Work out the finished part from the listing and answer in its coordinate system (mm). A direction names the side the tool comes from. Round coordinates to 2 decimals unless told otherwise and drop trailing zeros. Order: outer loops, then holes, each group sorted by start corner. A loop starts at its lowest first (then second) coordinate and runs counter-clockwise, first axis right, second up. Notation, with made-up numbers: (77.25, -25.5) - (88.25, -25.5) arc R10 ccw to (88.25, -13.5) - close; hole circle Ø9 at (-20.75, -26.75). An arc over 180 degrees is marked (long way). Use CSV: the item, a comma, the result in double quotes.
from build123d import *

# Parameters (mm, degrees)
SKETCH_1_W               = 25
SKETCH_1_H               = 16
EXTRUDE_1_DEPTH          = 7
SKETCH_3_W               = 5.9
SKETCH_3_H               = 2.3
FILLET_1_R               = 2
SKETCH_4_R               = 1.75
CUT_EXTRUDE_1_DEPTH      = 37.390245946
CUT_EXTRUDE_2_DEPTH      = 4.5
PATTERN_CIRCULAR_1_COUNT = 18


with BuildPart() as part:
    # 草图1 → 凸台-拉伸1 (new, symmetric)
    with BuildSketch(Plane(origin=(0, 0, 0), x_dir=(1, 0, 0), z_dir=(0, 1, 0))):
        Rectangle(SKETCH_1_W, SKETCH_1_H)
    extrude(amount=EXTRUDE_1_DEPTH, both=True)

    # 草图2 → 旋转1 (revolve)
    with BuildSketch(Plane(origin=(0, 0, 0), x_dir=(1, 0, 0), z_dir=(0, 1, 0)), mode=Mode.PRIVATE) as revolve_1_sk:
        Polygon((-12.5, 4.975068019), (-18.5, 5.5), (-21.5, 5.5), (-21.5, 4.5), (-22.5, 4.5), (-22.5, 6), (-24, 6), (-24, 3), (-19.5, 3), (-19.5, 2), (-12.5, 2), align=None)
        Polygon((19.5, 2), (12.5, 2), (12.5, 4.975068019), (18.5, 5.5), (21.5, 5.5), (21.5, 4.5), (22.5, 4.5), (22.5, 6), (24, 6), (24, 3), (19.5, 3), align=None)
    revolve(revolve_1_sk.sketch.rotate(Axis((-27.060600163, 0, 0), (1, 0, 0)), 180), axis=Axis((-27.060600163, 0, 0), (1, 0, 0)))

    # 草图3 → 旋转2 (revolve)
    with BuildSketch(Plane(origin=(0, 0, 0), x_dir=(1, 0, 0), z_dir=(0, 1, 0))):
        Polygon((7, 8), (7, 10.5), (6.5, 11), (6.5, 12.5), (4, 12.5), (4, 13.5), (4.4, 13.5), (4.4, 16), (2, 16), (2, 19), (4, 19), (4, 23.5), (0, 23.5), (0, 8), align=None)
        with Locations((2.95, -9.15)):
            Rectangle(SKETCH_3_W, SKETCH_3_H)
    revolve(axis=Axis((0, 0, 30.021655922), (0, 0, -1)))

    # 圆角1
    fillet_1_edges = [part.edges().sort_by_distance(p)[0] for p in [
        (-12.5, 0, -8),
        (12.5, 0, -8),
    ]]
    fillet(fillet_1_edges, radius=FILLET_1_R)

    # 草图4 → 切除-拉伸1 (cut, through all)
    with BuildSketch(Plane(origin=(0, 7, 0), x_dir=(1, 0, 0), z_dir=(0, 1, 0))):
        with Locations(Location((-10, 5.5, 0), (0, 0, 270))):
            Circle(SKETCH_4_R)
        with Locations(Location((10, 5.5, 0), (0, 0, 270))):
            Circle(SKETCH_4_R)
    extrude(amount=-CUT_EXTRUDE_1_DEPTH, mode=Mode.SUBTRACT)

    # 草图5 → 切除-拉伸2 (cut)
    with BuildSketch(Plane(origin=(0, 0, -23.5), x_dir=(-1, 0, 0), z_dir=(0, 0, -1))):
        with BuildLine():
            ThreePointArc((0, 4), (0.352895639, 3.937075737), (0.662294506, 3.756058788))
            ThreePointArc((0.662294506, 3.756058788), (1.01494578, 3.820338434), (1.368080573, 3.758770483))
            ThreePointArc((1.368080573, 3.758770483), (0.694592711, 3.939231012), (0, 4))
        make_face()
    cut_extrude_2 = extrude(amount=-CUT_EXTRUDE_2_DEPTH, mode=Mode.SUBTRACT)

    # 阵列(圆周)1: 切除-拉伸2 ×18 about axis
    pattern_circular_1_axis = Axis((0, 0, 0), (0, 0, 1))
    for i in range(1, PATTERN_CIRCULAR_1_COUNT):
        add(cut_extrude_2.rotate(pattern_circular_1_axis, i * 360 / PATTERN_CIRCULAR_1_COUNT), mode=Mode.SUBTRACT)


solid = part.part
(1) Find the intervals of material crossed by L1, parallel to X at y = -3.25, z = -5.5; L2, parallel to X at y = 1, z = -5.5; L3, parallel to X at y = 2.25, z = -7, in increasing order. Write a range as from..to.
Findings below:
L1,"x = -12.5..-11.75, -8.25..8.25, 11.75..12.5"
L2,"x = -24..-22.5, -12.5..-11.75, -8.25..8.25, 11.75..12.5, 22.5..24"
L3,"x = -12.23..-10.9, -9.1..9.1, 10.9..12.23"
(2) Each of these flat-tipped pins is pushed along its axis until it touches: pin 1 (4.5 mm diameter, centred on y = 0, z = 0, fed in from +X); pin 2 (4 mm diameter, centred on y = 0, z = 0.5, fed in from -X); pin 3 (5 mm diameter, centred on y = -2, z = -18, fed in from -X); pin 4 (4 mm diameter, centred on x = 16.5, z = -8, fed in from -Y). Where does it stop, or does it pass through?
Findings below:
pin 1,"stops at x = 19.5"
pin 2,"stops at x = -19.5"
pin 3,"stops at x = -4.37"
pin 4,"passes through"
(3) For faces 1 (the cylindrical face through (4.197, -1.322, -14.768)), 2 (the conical face through (-14.875, 3.154, -4.113)), 3 (the flat face through (19.5, 2, 1)), determine the directions among +Z, -Z, +X, -X, +Y, -Y from which every point of the face is accessible in a straight line to the end or side of a thin tool.
Findings below:
face 1,"-Z"
face 2,"none"
face 3,"+X"
(4) Find section D-D (x = 20). Determine the outline of the cut face in (y, z), and give its area (3 significant figures).
Findings below:
outline,"circle Ø11 at (0, 0); hole circle Ø6 at (0, 0)"
area,"66.8 mm²"
(5) Find section A-A (x = 10). Determine the outline of the cut face in (y, z).
Findings below:
outline,"(-7, -8) - (7, -8) - (7, -7.25) - (-7, -7.25) - close; (-7, -3.75) - (7, -3.75) - (7, 8) - (-7, 8) - close"
(6) The mould has two halves that part along Y. Classify faces 4 (the cylindrical face through (-5.158, 3.955, -11.76)), 5 (the flat face through (-12.5, 0, 0)), 6 (the flat face through (0, 7, 0)): released by +Y, released by -Y, zero draft, split by the parting line, or undercut.
Findings below:
face 4,"split by the parting line"
face 5,"undercut"
face 6,"released by +Y"
(7) Find section C-C (z = -12). Determine the outline of the cut face in (x, y), and give its area (3 significant figures).
Findings below:
outline,"circle Ø13 at (0, 0)"
area,"133 mm²"
(8) Find section B-B (y = -5). State how many separate pieces and enclosed holes the cut face has, and give its area (3 significant figures).
Findings below:
separate pieces,"5"
enclosed holes,"2"
area,"517 mm²"
